```python
from build123d import *

# Parameters (mm, degrees)
F0_R     = 31.75
F0_R_2   = 3.175
F1_DEPTH = 9.525
F2_R     = 31.75
F2_R_2   = 29.765094
F3_DEPTH = 6.35
F4_R     = 3.175
F5_DEPTH = 9.526
F6_W     = 6.35
F6_H     = 12.7
F7_DEPTH = 25.4
F8_W     = 9.525
F8_H     = 15.875
F9_DEPTH = 1.5748
F10_R    = 0.635


with BuildPart() as f1:
    # F0 (on Top) → F1 (new body)
    with BuildSketch(Plane.XY):
        Circle(F0_R)
        with Locations((0, -25.4)):
            Circle(F0_R_2, mode=Mode.SUBTRACT)
        with Locations((-25.4, 0)):
            Circle(F0_R_2, mode=Mode.SUBTRACT)
        with Locations((25.4, 0)):
            Circle(F0_R_2, mode=Mode.SUBTRACT)
        with Locations((0, 25.4)):
            Circle(F0_R_2, mode=Mode.SUBTRACT)
    extrude(amount=F1_DEPTH)

    # F2 (on face) → F3 (cut)
    with BuildSketch(Plane(origin=(0, 0, 0), x_dir=(1, 0, 0), z_dir=(0, 0, -1))):
        Circle(F2_R)
        Circle(F2_R_2, mode=Mode.SUBTRACT)
    extrude(amount=-F3_DEPTH, mode=Mode.SUBTRACT)

    # F4 (on face) → F5 (cut, through all)
    with BuildSketch(Plane(origin=(0, 0, 0), x_dir=(1, 0, 0), z_dir=(0, 0, -1))):
        Circle(F4_R)
    extrude(amount=-F5_DEPTH, mode=Mode.SUBTRACT)

    # F6 (on face) → F7 (cut)
    with BuildSketch(Plane(origin=(0, 0, 0), x_dir=(1, 0, 0), z_dir=(0, 0, -1))):
        with Locations((16.909514, 0)):
            Rectangle(F6_W, F6_H)
    extrude(amount=-F7_DEPTH, mode=Mode.SUBTRACT)

    # F8 (on face) → F9 (cut)
    with BuildSketch(Plane.XY.offset(9.525)):
        with Locations((16.939783, 0)):
            Rectangle(F8_W, F8_H)
    extrude(amount=-F9_DEPTH, mode=Mode.SUBTRACT)

    # F10
    f10_edges = [f1.edges().sort_by_distance(p)[0] for p in [
        (13.734514, -6.35, 3.9751),
        (13.734514, 6.35, 3.9751),
        (20.084514, -6.35, 3.9751),
        (20.084514, 6.35, 3.9751),
        (21.702283, 7.9375, 8.7376),
        (21.702283, -7.9375, 8.7376),
        (12.177283, -7.9375, 8.7376),
        (12.177283, 7.9375, 8.7376),
    ]]
    fillet(f10_edges, radius=F10_R)


solid = f1.part
```
Read the model definition and answer for the solid it produces. Units are mm, in the model's axes. A direction names the side the tool comes from. Give positions to 0.01 mm unless a question says otherwise; leave off trailing zeros. Write each loop counter-clockwise with the first axis right and the second up, starting at its lowest first coordinate (ties: lowest second). Pieces come first, ordered by that corner, then holes. Notation, with made-up numbers: (27, 35.5) -> (82, 35.5) arc R15 cw to (82, 48.5) -> close; hole circle Ø5 at (59, 87). An arc over 180 degrees is marked (long way). Answer as a JSON object with one key per item and string values.
1) Section C-C on y = 1 is taken. Write down the section's boundary in (x, z) (3 decimals), then the cut area to 3 significant figures.
Findings below:
{"outline": "(-31.734, 6.35) -> (-29.748, 6.35) -> (-29.748, 0) -> (-28.413, 0) -> (-28.413, 9.525) -> (-31.734, 9.525) -> close; (-22.387, 0) -> (-3.013, 0) -> (-3.013, 9.525) -> (-22.387, 9.525) -> close; (3.013, 0) -> (13.735, 0) -> (13.735, 7.95) -> (12.177, 7.95) -> (12.177, 9.525) -> (3.013, 9.525) -> close; (20.085, 0) -> (22.387, 0) -> (22.387, 9.525) -> (21.702, 9.525) -> (21.702, 7.95) -> (20.085, 7.95) -> close; (28.413, 0) -> (29.748, 0) -> (29.748, 6.35) -> (31.734, 6.35) -> (31.734, 9.525) -> (28.413, 9.525) -> close", "area": "342 mm^2"}
2) Section A-A on z = 1.5 is taken. Write down the section's boundary in (x, y) (3 decimals).
Findings below:
{"outline": "circle Ø59.53 at (0, 0); hole circle Ø6.35 at (-25.4, 0); hole circle Ø6.35 at (0, -25.4); hole circle Ø6.35 at (0, 0); hole circle Ø6.35 at (0, 25.4); hole (13.735, -5.715) arc R0.635 ccw to (14.37, -6.35) -> (19.45, -6.35) arc R0.635 ccw to (20.085, -5.715) -> (20.085, 5.715) arc R0.635 ccw to (19.45, 6.35) -> (14.37, 6.35) arc R0.635 ccw to (13.735, 5.715) -> close; hole circle Ø6.35 at (25.4, 0)"}
3) For a pull along X with two mould halves and no side action, classify faces 1 (the flat face through (0, -6, 0)), 2 (the cylindrical face through (-22.37, 0.95, 4.7)), 3 (the cylindrical face through (-6.883, -30.995, 7.915)) as pulls with the +X half, pulls with the -X half, needs draft (parallel to the pull), parting line crosses it, or undercut.
Findings below:
{"face 1": "needs draft", "face 2": "undercut", "face 3": "parting line crosses it"}
4) Straight lines are drawn through the part: probe 1 along Y at (x, z) = (0, 3.5) (3 decimals); probe 2 along Y at (x, z) = (0, 7.25) (3 decimals); probe 3 along Y at (x, z) = (-26.5, 8.75). For each, find the intervals that lie inside material, in ascending order. Write a range as from..to.
Findings below:
{"probe 1": "y = -29.765..-28.575, -22.225..-3.175, 3.175..22.225, 28.575..29.765", "probe 2": "y = -31.75..-28.575, -22.225..-3.175, 3.175..22.225, 28.575..31.75", "probe 3": "y = -17.49..-2.98, 2.98..17.49"}
5) Flat-ended cylindrical pins translate along their axes: pin 1 Ø1.7 at (y, z) = (-3, 8.5) entering from +X; pin 2 Ø1 at (x, z) = (-4.5, 3.5) entering from +Y; pin 3 Ø1.3 at (x, z) = (18, 9) entering from -Y. Find the tip coordinate at first contact, or state that the pin passes through.
Findings below:
{"pin 1": "stops at x = 31.68", "pin 2": "stops at y = 29.5", "pin 3": "stops at y = -26.59"}
6) A tool of negligible diameter and unlimited length cuts with its end or side. For faces 4 (the flat face through (13.735, 0, 4)), 5 (the flat face through (-9.6, -28.4, 6.35)), 6 (the flat face through (12.177, 0, 9)), from which of +Z, -Z, +X, -X, +Y, -Y can it reach the whole face along a straight path? Write none if from no direction.
Findings below:
{"face 4": "+Z, -Z", "face 5": "-Z", "face 6": "+Z"}
7) Section D-D on x = -25.4 is taken. Write down the section's boundary in (y, z) (3 decimals), then the cut area to 3 significant figures.
Findings below:
{"outline": "(-19.05, 6.35) -> (-15.518, 6.35) -> (-15.518, 0) -> (-3.175, 0) -> (-3.175, 9.525) -> (-19.05, 9.525) -> close; (3.175, 0) -> (15.518, 0) -> (15.518, 6.35) -> (19.05, 6.35) -> (19.05, 9.525) -> (3.175, 9.525) -> close", "area": "258 mm^2"}
8) Section B-B on x = 0 is taken. Write down the section's boundary in (y, z) (3 decimals), then the cut area to 3 significant figures.
Findings below:
{"outline": "(-31.75, 6.35) -> (-29.765, 6.35) -> (-29.765, 0) -> (-28.575, 0) -> (-28.575, 9.525) -> (-31.75, 9.525) -> close; (-22.225, 0) -> (-3.175, 0) -> (-3.175, 9.525) -> (-22.225, 9.525) -> close; (3.175, 0) -> (22.225, 0) -> (22.225, 9.525) -> (3.175, 9.525) -> close; (28.575, 0) -> (29.765, 0) -> (29.765, 6.35) -> (31.75, 6.35) -> (31.75, 9.525) -> (28.575, 9.525) -> close", "area": "398 mm^2"}
